Source: CAD feature listing. Evaluate the final solid. Frame: model axes, mm. A direction names the side the tool comes from. Give positions to 0.01 mm unless a question says otherwise; leave off trailing zeros. Write each loop counter-clockwise with the first axis right and the second up, starting at its lowest first coordinate (ties: lowest second). Pieces come first, ordered by that corner, then holes.
```python
from build123d import *

# Parameters (mm, degrees)
SALIENTE_EXTRUIR2_DEPTH = 76.2
CORTAR_EXTRUIR3_START   = -25.4
CORTAR_EXTRUIR3_DEPTH   = 25.4


with BuildPart() as part:
    # Croquis2 → Saliente-Extruir2 (new body)
    with BuildSketch(Plane(origin=(0, 0, 0), x_dir=(0, 0, -1), z_dir=(1, 0, 0))):
        Polygon((0, 0), (38.1, 0), (38.1, 50.8), (12.7, 50.8), (0, 25.4), (-12.7, 25.4), (-12.7, 12.7), align=None)
    extrude(amount=SALIENTE_EXTRUIR2_DEPTH)

    # Croquis4 → Cortar-Extruir3 (cut)
    with BuildSketch(Plane(origin=(76.2, 0, 0), x_dir=(0, 0, -1), z_dir=(1, 0, 0)).offset(CORTAR_EXTRUIR3_START)):
        Polygon((0, 25.4), (38.1, 50.8), (12.7, 50.8), align=None)
    extrude(amount=-CORTAR_EXTRUIR3_DEPTH, mode=Mode.SUBTRACT)


solid = part.part
```
1. Access query for faces 1 (the flat face through (50.8, 41, -19)), 2 (the flat face through (38, 0, -19)), 3 (the flat face through (38, 25.4, 6)). Directions: +Z, -Z, +X, -X, +Y, -Y. A direction counts if a zero-diameter tool reaches every point of the face in a straight line with its end or side. Return the directions, or none.
2. Section query A-A (y = 40). Return loops of the section in (x, z).
3. Line query: probe 1 along X at (y, z) = (35.5, -13); probe 2 along Z at (x, y) = (71.5, 27); probe 3 along Y at (x, z) = (44.5, -24). Output: solid intervals per line, ascending.
4. Pull-direction query (X, two-part tool) for faces 4 (the flat face through (76.2, 26, -18)), 5 (the flat face through (0, 26, -18)), 6 (the flat face through (25.4, 41, -19)), 7 (the flat face through (63, 50.8, -26)); classes: pulls with the +X half, pulls with the -X half, needs draft (parallel to the pull), parting line crosses it, or undercut.
5. Section query C-C (z = -31.5). Return loops of the section in (x, y), plus the area to 3 significant figures.
6. Pin query (flat end, axial travel): P1, Ø6, axis at y = 36.5, z = -1.5, coming from the -X side; P2, Ø6, axis at x = 51, z = 7.5, coming from the +Y side; P3, Ø14, axis at x = 51.5, z = 4.5, coming from the +Y side; P4, Ø2, axis at x = 29, z = 4, coming from the -Y side. Return the tip coordinate at first contact, or that it passes through.
7. Section query D-D (x = 35.5). Return loops of the section in (y, z), plus the area to 3 significant figures.
8. Section query B-B (x = 10). Return loops of the section in (y, z).
The answers:
1. face 1: +Z, +Y
1. face 2: +Z, -Z, +X, -X, -Y
1. face 3: +Z, +X, -X, +Y
2. outline: (0, -38.1) - (76.2, -38.1) - (76.2, -7.3) - (50.8, -7.3) - (50.8, -21.9) - (25.4, -21.9) - (25.4, -7.3) - (0, -7.3) - close
3. probe 1: x = 0 to 25.4, 50.8 to 76.2
3. probe 2: z = -38.1 to -0.8
3. probe 3: y = 0 to 41.4
4. face 4: pulls with the +X half
4. face 5: pulls with the -X half
4. face 6: undercut
4. face 7: needs draft
5. outline: (0, 0) - (76.2, 0) - (76.2, 50.8) - (50.8, 50.8) - (50.8, 46.4) - (25.4, 46.4) - (25.4, 50.8) - (0, 50.8) - close
5. area: 3,760 mm2
6. P1: passes through
6. P2: stops at y = 25.4
6. P3: stops at y = 30.4
6. P4: stops at y = 3
7. outline: (0, -38.1) - (50.8, -38.1) - (25.4, 0) - (25.4, 12.7) - (12.7, 12.7) - (0, 0) - close
7. area: 1,690 mm2
8. outline: (0, -38.1) - (50.8, -38.1) - (50.8, -12.7) - (25.4, 0) - (25.4, 12.7) - (12.7, 12.7) - (0, 0) - close
